```python
from build123d import *

# Parameters (mm, degrees)
SKETCH1_R           = 8
BOSS_EXTRUDE1_DEPTH = 2
CHAMFER1_SIZE       = 1
SKETCH2_R           = 2.5
CUT_EXTRUDE1_DEPTH  = 2


with BuildPart() as part:
    # Sketch1 → Boss-Extrude1 (new body)
    with BuildSketch(Plane(origin=(0, 0, 0), x_dir=(1, 0, 0), z_dir=(0, 1, 0))):
        Circle(SKETCH1_R)
    extrude(amount=BOSS_EXTRUDE1_DEPTH)

    # Chamfer1
    chamfer1_edges = [part.edges().sort_by_distance(p)[0] for p in [
        (-8, 2, 0),
    ]]
    chamfer(chamfer1_edges, length=CHAMFER1_SIZE)

    # Sketch2 → Cut-Extrude1 (cut)
    with BuildSketch(Plane(origin=(0, 2, 0), x_dir=(1, 0, 0), z_dir=(0, 1, 0))):
        Circle(SKETCH2_R)
    extrude(amount=-CUT_EXTRUDE1_DEPTH, mode=Mode.SUBTRACT)


solid = part.part
```
Geometry: final body of the model. Coordinates: model frame, mm. Round coordinates to 2 decimals unless told otherwise and drop trailing zeros. Loops run counter-clockwise (first coordinate to the right, second up) from the corner with the lowest first, then second, coordinate; pieces in that order, holes last. Notation, with made-up numbers: (39, -26.5) -> (46, -26.5) arc R27 ccw to (46, 12.5) -> close; hole circle Ø5 at (-7, 67). An arc over 180 degrees is marked (long way). Use one line per item in the form item = value. Start each with the question number.
1) Section A-A on x = 0. Output: boundary loops of the cut face in (y, z).
2) Draft query along Z for faces 1 (the flat face through (2, 0, -2)), 2 (the cylindrical face through (-1.73, 0.49, 7.81)), 3 (the cylindrical face through (-0.54, 1.01, 2.44)). Return one class per face: released by +Z, released by -Z, zero draft, split by the parting line, or undercut.
3) Section B-B on z = 0. Output: boundary loops of the cut face in (x, y), then the cut area to 3 significant figures.
4) Section D-D on y = 0.6. Output: boundary loops of the cut face in (x, z), then the cut area to 3 significant figures.
5) Section C-C on y = 1.8. Output: boundary loops of the cut face in (x, z).
6) Line query: L1, parallel to Z at x = 0, y = 0.65; L2, parallel to X at y = 1.4, z = 0. Output: solid intervals per line, ascending.
Response:
q1.outline = (0, -8) -> (1, -8) -> (2, -7) -> (2, -2.5) -> (0, -2.5) -> close; (0, 2.5) -> (2, 2.5) -> (2, 7) -> (1, 8) -> (0, 8) -> close
q2.face_1 = zero draft
q2.face_2 = split by the parting line
q2.face_3 = undercut
q3.outline = (-8, 0) -> (-2.5, 0) -> (-2.5, 2) -> (-7, 2) -> (-8, 1) -> close; (2.5, 0) -> (8, 0) -> (8, 1) -> (7, 2) -> (2.5, 2) -> close
q3.area = 21.0 mm^2
q4.outline = circle Ø16 at (0, 0); hole circle Ø5 at (0, 0)
q4.area = 181 mm^2
q5.outline = circle Ø14.4 at (0, 0); hole circle Ø5 at (0, 0)
q6.L1 = -8 to -2.5, 2.5 to 8
q6.L2 = -7.6 to -2.5, 2.5 to 7.6
